Source: three-view drawing plus pictorial views. Frame: mm from the lowest corner of the part. A direction names the side the tool comes from. Give positions to 0.01 mm unless a question says otherwise; leave off trailing zeros. Write each loop counter-clockwise with the first axis right and the second up, starting at its lowest first coordinate (ties: lowest second). Pieces come first, ordered by that corner, then holes.
Q1. Pin query (flat end, axial travel): pin 1 (12 mm diameter, centred on x = 13.5, y = 25.5, fed in from +Z); pin 2 (2 mm diameter, centred on x = 21, y = 10, fed in from +Z); pin 3 (6 mm diameter, centred on y = 8, z = 57, fed in from +X). Return the tip coordinate at first contact, or that it passes through.
Q2. Cut plane C-C on z = 58. Return the cut outline in (x, y).
Q3. Cut plane B-B on y = 18.5. Return the cut outline in (x, z).
Q4. Draft query along X for the marked faces 4, 5, 6 and 7. Return one class per face: pulls with the +X half, pulls with the -X half, needs draft (parallel to the pull), parting line crosses it, or undercut.
Q5. Cut plane A-A on x = 18.5. Return the cut outline in (y, z), plus the area to 3 significant figures.
Q6. Cut plane D-D on y = 24. Return the cut outline in (x, z) (1 decimal).
Q7. Line query: L1, parallel to Z at x = 29, y = 18.5; L2, parallel to Y at x = 18.5, z = 40.75; L3, parallel to Z at x = 30.5, y = 6.5. Output: solid intervals per line, ascending.
Q8. Reachability of the marked faces 1, 2 and 3 from +Z, -Z, +X, -X, +Y, -Y: full face, straight path, thin tool, end or side. Return the list, or none.
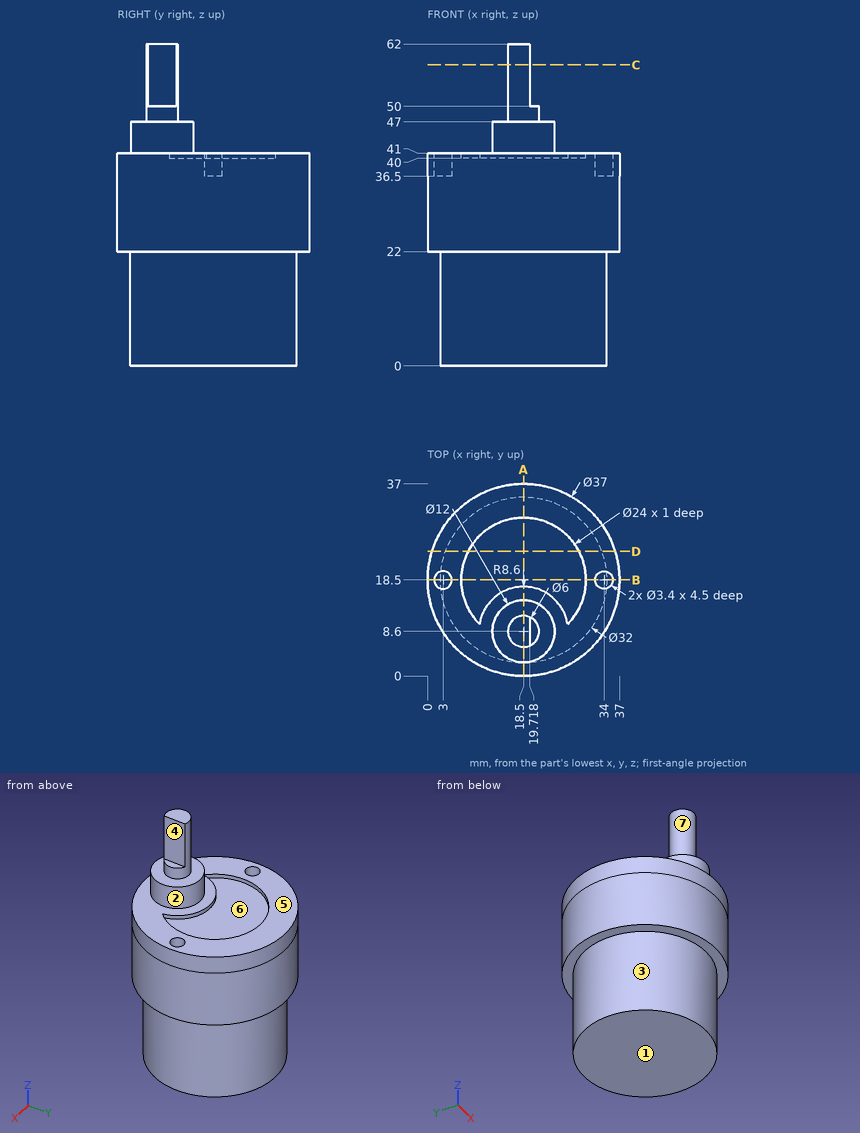
Data:
1. pin 1: stops at z = 41
1. pin 2: stops at z = 50
1. pin 3: stops at x = 19.72
2. outline: (19.72, 5.86) - (19.72, 11.34) arc R3 ccw (long way) to start
3. outline: (0, 22) - (2.5, 22) - (2.5, 0) - (34.5, 0) - (34.5, 22) - (37, 22) - (37, 41) - (35.7, 41) - (35.7, 36.5) - (32.3, 36.5) - (32.3, 41) - (30.5, 41) - (30.5, 40) - (6.5, 40) - (6.5, 41) - (4.7, 41) - (4.7, 36.5) - (1.3, 36.5) - (1.3, 41) - (0, 41) - close
4. face 4: pulls with the +X half
4. face 5: needs draft
4. face 6: undercut
4. face 7: parting line crosses it
5. outline: (0, 22) - (2.5, 22) - (2.5, 0) - (34.5, 0) - (34.5, 22) - (37, 22) - (37, 41) - (30.5, 41) - (30.5, 40) - (17.2, 40) - (17.2, 41) - (14.6, 41) - (14.6, 47) - (11.6, 47) - (11.6, 62) - (5.6, 62) - (5.6, 47) - (2.6, 47) - (2.6, 41) - (0, 41) - close
5. area: 1,560 mm2
6. outline: (0.8, 22) - (3.5, 22) - (3.5, 0) - (33.5, 0) - (33.5, 22) - (36.2, 22) - (36.2, 41) - (29.2, 41) - (29.2, 40) - (7.8, 40) - (7.8, 41) - (0.8, 41) - close
7. L1: z = 0 to 40
7. L2: y = 0 to 17.2, 30.5 to 37
7. L3: z = 22 to 41
8. face 1: -Z, +X, -X, +Y, -Y
8. face 2: +Z
8. face 3: -Z
